Part model, mm, in its own coordinate system. A direction names the side the tool comes from. Give positions to 0.01 mm unless a question says otherwise; leave off trailing zeros. Write each loop counter-clockwise with the first axis right and the second up, starting at its lowest first coordinate (ties: lowest second). Pieces come first, ordered by that corner, then holes.
```python
from build123d import *

# Parameters (mm, degrees)
PAD_DEPTH       = 20
SKETCH001_R     = 2.5
POCKET_DEPTH    = 25.001
POCKET001_DEPTH = 5.5
POCKET002_DEPTH = 5.5
SKETCH004_W     = 4.5
SKETCH004_H     = 4.5
PAD001_DEPTH    = 5


with BuildPart() as part:
    # Sketch → Pad (new body)
    with BuildSketch(Plane.XZ):
        Polygon((0, 0), (20, 0), (20, 15), (-5, 15), (-5, -10), (0, -10), align=None)
    extrude(amount=PAD_DEPTH)

    # Sketch001 (on Face3 of Pad) → Pocket (cut, through all)
    with BuildSketch(Plane(origin=(0, 0, 15), x_dir=(-1, 0, 0), z_dir=(0, 0, 1))):
        with Locations((-10.5, 10)):
            Circle(SKETCH001_R)
    extrude(amount=-POCKET_DEPTH, mode=Mode.SUBTRACT)

    # Sketch002 (on Face8 of Pocket) → Pocket001 (cut)
    with BuildSketch(Plane(origin=(0, 0, 15), x_dir=(-1, 0, 0), z_dir=(0, 0, 1))):
        Polygon((-8.190599, 14), (-12.809401, 14), (-15.118802, 10), (-12.809401, 6), (-8.190599, 6), (-5.881198, 10), align=None)
    extrude(amount=-POCKET001_DEPTH, mode=Mode.SUBTRACT)

    # Sketch003 (on Face1 of Pocket001) → Pocket002 (cut)
    with BuildSketch(Plane(origin=(0, 0, 0), x_dir=(1, 0, 0), z_dir=(0, 0, -1))):
        Polygon((10.5, 14.618802), (6.5, 12.309401), (6.5, 7.690599), (10.5, 5.381198), (14.5, 7.690599), (14.5, 12.309401), align=None)
    extrude(amount=-POCKET002_DEPTH, mode=Mode.SUBTRACT)

    # Sketch004 (on Face1 of Pocket002) → Pad001 (join)
    with BuildSketch(Plane(origin=(0, 0, 0), x_dir=(1, 0, 0), z_dir=(0, 0, -1))):
        with Locations((2.25, 10)):
            Rectangle(SKETCH004_W, SKETCH004_H)
    extrude(amount=PAD001_DEPTH)


solid = part.part
```
1) 3-axis set-ups, long thin cutter, end or side, ignore diameter. For faces 1 (the face through (7.02, -11.97, 12.29)), 2 (the face through (4.5, -10, -2)), 3 (the face through (12.47, -6.52, 2.71)): which of +Z, -Z, +X, -X, +Y, -Y reach the whole face in a straight line?
Answers follow:
face 1: +Z
face 2: -Z, +X, +Y, -Y
face 3: -Z
2) Saw through at A-A, the plane x = 0.5. Write the cut outline in (y, z).
Answers follow:
outline: (-20, 0) - (-12.25, 0) - (-12.25, -5) - (-7.75, -5) - (-7.75, 0) - (0, 0) - (0, 15) - (-20, 15) - close
3) Pin check, flat tips, straight feed: pin 1 Ø4 at (x, z) = (2.5, -5.5) entering from -Y; pin 2 Ø6.5 at (x, y) = (12.5, -11.5) entering from -Z; pin 3 Ø3 at (y, z) = (-13.5, -7.5) entering from +X; pin 4 Ø4.5 at (x, y) = (10.5, -10) entering from +Z. Stop position of each tip, or through.
Answers follow:
pin 1: stops at y = -12.25
pin 2: stops at z = 0
pin 3: stops at x = 0
pin 4: passes through
4) Wall check: L1, parallel to X at y = -10, z = 8.2; L2, parallel to Y at x = 10.25, z = 11.5; L3, parallel to Y at x = 10.5, z = 7.3. Give the ranges that are in metal, low to high.
Answers follow:
L1: x = -5 to 8, 13 to 20
L2: y = -20 to -14, -6 to 0
L3: y = -20 to -12.5, -7.5 to 0
5) Saw through at D-D, the plane y = -18. Write the cut outline in (x, z), then the cut area to 3 significant figures.
Answers follow:
outline: (-5, -10) - (0, -10) - (0, 0) - (20, 0) - (20, 15) - (-5, 15) - close
area: 425 mm2
6) Saw through at C-C, the plane y = -11.75. Write the cut outline in (x, z), then the cut area to 3 significant figures.
Answers follow:
outline: (-5, -10) - (0, -10) - (0, -5) - (4.5, -5) - (4.5, 0) - (6.5, 0) - (6.5, 5.5) - (8.71, 5.5) - (8.71, 9.5) - (6.89, 9.5) - (6.89, 15) - (-5, 15) - close; (12.29, 5.5) - (14.5, 5.5) - (14.5, 0) - (20, 0) - (20, 15) - (14.11, 15) - (14.11, 9.5) - (12.29, 9.5) - close
area: 350 mm2
7) Saw through at B-B, the plane z = 12.5. Write the cut outline in (x, y), then the cut area to 3 significant figures.
Answers follow:
outline: (-5, -20) - (20, -20) - (20, 0) - (-5, 0) - close; hole (5.88, -10) - (8.19, -14) - (12.81, -14) - (15.12, -10) - (12.81, -6) - (8.19, -6) - close
area: 445 mm2
